Autodesk Inventor part; units mm, degrees
ref_plane "YZ Plane" through (0, 0, 0) normal (1, 0, 0) x (0, 1, 0)
ref_plane "XZ Plane" through (0, 0, 0) normal (0, 1, 0) x (-1, 0, 0)
ref_plane "XY Plane" through (0, 0, 0) normal (0, 0, 1) x (1, 0, 0)
sketch "Sketch1" plane through (0, 0, 0) normal (0, 0, 1) x (1, 0, 0)
  line L0 (0, 0) -> (50.8, 0)
  line L1 (50.8, 0) -> (50.8, 25.4)
  line L2 (50.8, 25.4) -> (0, 25.4)
  line L3 (0, 25.4) -> (0, 0)
  line L4 (3.175, 22.225) -> (47.625, 22.225)
  line L5 (47.625, 22.225) -> (47.625, 3.175)
  line L6 (47.625, 3.175) -> (3.175, 3.175)
  line L7 (3.175, 3.175) -> (3.175, 22.225)
  dimension "d0" = 50.8
  dimension "d1" = 25.4
  dimension "d2" = 3.175
extrude "Extrusion1" add sketch "Sketch1" along normal blind 254
sketch "Sketch2" plane through (0, 0, 0) normal (0, -1, 0) x (1, 0, 0)
  circle A0 centre (25.4, 228.6) radius 4.7625
  line L0 (47.625, 254) -> (3.175, 254)
  line L1 (0, 0) -> (0, 254)
  dimension "d5" = 9.525
  dimension "d6" = 25.4
  dimension "d7" = 25.4
extrude "Extrusion2" cut sketch "Sketch2" against normal blind 25.4
sketch "Sketch3" plane through (0, 25.4, 0) normal (0, 1, 0) x (1, 0, 0)
  circle A0 centre (25.4, -228.6) radius 4.7625
  circle A1 centre (25.4, -228.6) radius 14.2875
  point P0 (0, 0)
  dimension "d10" = 28.575
extrude "Extrusion3" cut sketch "Sketch3" against normal blind 25.4
ref_plane "Work Plane1" through (25.4, 0, 228.6) normal (0, 0, -1) x (1, 0, 0)
sketch "Sketch5" plane through (50.8, 0, 0) normal (1, 0, 0) x (0, 0, -1)
  line L0 (-254, 0) -> (-254, 25.4)
  line L1 (0, 0) -> (-254, 0)
  line L2 (0, 25.4) -> (-254, 25.4)
  point P0 (-228.6, 12.7)
  point P1 (-203.2, 12.7)
  point P2 (-177.8, 12.7)
  dimension "d21" = 25.4
  dimension "d22" = 12.7
  dimension "d23" = 25.4
  dimension "d24" = 25.4
  dimension "d25" = 12.7
  dimension "d26" = 12.7
hole "Hole1" at (50.8, 12.7, 228.6) at (50.8, 12.7, 203.2) at (50.8, 12.7, 177.8) direction (-1, 0, 0) diameter 5.1594 end through all
thread "Thread1"
thread "Thread2"
thread "Thread3"
properties part number "15102898-16-A-0201" material "Aluminum 6061"
Read the model definition and answer for the solid it produces. Units are mm, in the model's axes. A direction names the side the tool comes from. Round coordinates to 2 decimals unless told otherwise and drop trailing zeros. Write each loop counter-clockwise with the first axis right and the second up, starting at its lowest first coordinate (ties: lowest second). Pieces come first, ordered by that corner, then holes. Notation, with made-up numbers: (73, 38) - (129, 38) arc R27 ccw to (129, 74) - close; hole circle Ø1 at (77.25, 53). An arc over 180 degrees is marked (long way). One line per question, with ' | ' between items. Start each with the question number.
1. Section A-A (z = 177.8) is taken. Determine the outline of the cut face in (x, y) (3 decimals).
2. Section B-B (y = 12.7) is taken. Give the number of separate pieces and of enclosed holes in the cut face, and give its area (3 significant figures).
3. For faces 4 (the face through (26, 3.175, 125)), 5 (the face through (49.19, 10.957, 179.701)), determine the directions among +Z, -Z, +X, -X, +Y, -Y from which every point of the face is accessible in a straight line to the end or side of a thin tool.
4. Section D-D (z = 29.5) is taken. Determine the outline of the cut face in (x, y) (3 decimals).
5. Find the intervals of material crossed by probe 1 along Z at (x, y) = (49.75, 12.7); probe 2 along Y at (x, z) = (28, 132) (3 decimals); probe 3 along Y at (x, z) = (2.5, 177.8), in increasing order. Write a range as [from, to].
6. For a pull along Z with two mould halves and no side action, classify faces 1 (the face through (3.175, 13, 125)), 2 (the face through (25, 23, 254)), 3 (the face through (49.19, 10.957, 230.501)) as +Z half, -Z half, draft (parallel to the pull), parting line (faces both ways), or undercut.
7. Section C-C (x = 25.4) is taken. Determine the outline of the cut face in (y, z) (1 decimal), and give its area (3 significant figures).
Filled in:
1) outline: (0, 0) - (50.8, 0) - (50.8, 10.12) - (47.625, 10.12) - (47.625, 3.175) - (3.175, 3.175) - (3.175, 10.12) - (0, 10.12) - close; (0, 15.28) - (3.175, 15.28) - (3.175, 22.225) - (47.625, 22.225) - (47.625, 15.28) - (50.8, 15.28) - (50.8, 25.4) - (0, 25.4) - close
2) separate pieces: 8 | enclosed holes: 0 | area: 1,510 mm²
3) face 4: +Z, -Z | face 5: +X, -X
4) outline: (0, 0) - (50.8, 0) - (50.8, 25.4) - (0, 25.4) - close; hole (3.175, 3.175) - (47.625, 3.175) - (47.625, 22.225) - (3.175, 22.225) - close
5) probe 1: [0, 175.22], [180.38, 200.62], [205.78, 226.02], [231.18, 254] | probe 2: [0, 3.175], [22.225, 25.4] | probe 3: [0, 10.12], [15.28, 25.4]
6) face 1: draft | face 2: +Z half | face 3: undercut
7) outline: (0, 0) - (3.2, 0) - (3.2, 214.3) - (0, 214.3) - close; (0, 242.9) - (3.2, 242.9) - (3.2, 254) - (0, 254) - close; (22.2, 0) - (25.4, 0) - (25.4, 214.3) - (22.2, 214.3) - close; (22.2, 242.9) - (25.4, 242.9) - (25.4, 254) - (22.2, 254) - close | area: 1,430 mm²
